Autodesk Inventor part; units mm, degrees
ref_plane "YZ Plane" through (0, 0, 0) normal (1, 0, 0) x (0, 1, 0)
ref_plane "XZ Plane" through (0, 0, 0) normal (0, 1, 0) x (-1, 0, 0)
ref_plane "XY Plane" through (0, 0, 0) normal (0, 0, 1) x (1, 0, 0)
sketch "Sketch1" plane through (0, 0, 0) normal (0, 0, 1) x (1, 0, 0)
  line L0 (198.6992, 341.4095) -> (224.0992, 341.4095)
  line L1 (274.8992, 290.6095) -> (274.8992, 239.8095)
  line L2 (224.0992, 189.0095) -> (122.4992, 189.0095)
  line L3 (198.4116, 290.6095) -> (198.6992, 290.6095)
  line L4 (224.0992, 265.2095) -> (224.0992, 265.2095)
  line L5 (198.6992, 239.8095) -> (122.4992, 239.8095)
  line L6 (198.6992, 341.4095) -> (198.6992, 290.6095)
  line L7 (122.4992, 239.8095) -> (122.4992, 189.0095)
  arc A0 (224.0992, 265.2095) -> (198.6992, 290.6095) centre (198.6992, 265.2095) ccw
  arc A1 (198.6992, 239.8095) -> (224.0992, 265.2095) centre (198.6992, 265.2095) ccw
  arc A2 (274.8992, 290.6095) -> (224.0992, 341.4095) centre (224.0992, 290.6095) ccw
  arc A3 (224.0992, 189.0095) -> (274.8992, 239.8095) centre (224.0992, 239.8095) ccw
  circle A4 centre (143.7935, 214.4095) radius 12.7
  point P0 (0, 0)
  point P1 (274.8992, 341.4095)
  point P2 (274.8992, 189.0095)
  point P3 (274.8992, 265.2095)
  dimension "d0" = 50.8
  dimension "d1" = 50.8
  dimension "d2" = 50.8
  dimension "d3" = 50.8
  dimension "d6" = 152.4
  dimension "d7" = 25.4
  dimension "d8" = 25.4
  dimension "d9" = 50.8
  dimension "d12" = 25.4
extrude "Extrusion1" add sketch "Sketch1" along normal blind 6.35 draft -15 contours L0 A2 L1 A3 L2 L7 L5 A1 A0 L6 | A4
properties part number "hook"
Geometry: final body of the model. Coordinates: model frame, mm. Round coordinates to 2 decimals unless told otherwise and drop trailing zeros. Order: outer loops, then holes, each group sorted by start corner. A loop starts at its lowest first (then second) coordinate and runs counter-clockwise, first axis right, second up. Notation, with made-up numbers: M -36,83 L 6,83 A31 cw 6,117 Z; hole C -21.5,0.25 d3. An arc over 180 degrees is marked long. Use one line per item in the form item = value. Start each with the question number.
Q1. Mould query, pull axis Y, two halves, no side actions, for faces 1 (the face through (160.07, 238.97, 3.13)), 2 (the face through (199.538, 315.654, 3.131)), 3 (the face through (224.388, 264.644, 1.103)). Classes: +Y half, -Y half, draft (parallel to the pull), parting line (faces both ways), or undercut.
Q2. Material intervals for line 1 (X direction, y = 237, z = 2); line 2 (Y direction, x = 156, z = 3.5); line 3 (Y direction, x = 174.5, z = 0.5), sorted ascending. Write a range as [from, to].
Q3. Cut plane A-A (z = 3). Return loops of the section in (x, y).
Q4. Cut plane B-B (x = 137). Return loops of the section in (y, z).
Q5. Pin query (flat end, axial travel): pin 1 Ø1 at (x, z) = (173.5, 1.5) entering from +Y; pin 2 Ø2 at (x, z) = (256, 2.5) entering from +Y; pin 3 Ø2 at (x, z) = (147, 3) entering from +Y. Return the tip coordinate at first contact, or that it passes through.
Geometry results:
q1.face_1 = +Y half
q1.face_2 = draft
q1.face_3 = undercut
q2.line_1 = [123.04, 274.28]
q2.line_2 = [189.95, 238.87]
q2.line_3 = [189.14, 239.68]
q3.outline = M 123.3,189.81 L 224.1,189.81 A50 ccw 274.1,239.81 L 274.1,290.61 A50 ccw 224.1,340.61 L 199.5,340.61 L 199.5,291.4 A26.2 cw 198.7,239.01 L 123.3,239.01 Z
q4.outline = M 189.01,0 L 239.81,0 L 238.11,6.35 L 190.71,6.35 Z
q5.pin_1 = 239.54
q5.pin_2 = 330.15
q5.pin_3 = 239.27
